from build123d import *

# Parameters (mm, degrees)
CROQUIS1_W              = 250
CROQUIS1_H              = 20
SALIENTE_EXTRUIR1_DEPTH = 250
CROQUIS2_R              = 3.25
CORTAR_EXTRUIR1_DEPTH   = 281.223125384


with BuildPart() as part:
    # Croquis1 → Saliente-Extruir1 (new body)
    with BuildSketch(Plane(origin=(0, 0, 0), x_dir=(1, 0, 0), z_dir=(0, 1, 0))):
        with Locations((0, 185.6)):
            Rectangle(CROQUIS1_W, CROQUIS1_H)
    extrude(amount=SALIENTE_EXTRUIR1_DEPTH)

    # Croquis2 → Cortar-Extruir1 (cut, through all)
    with BuildSketch(Plane.XY.offset(-175.6)):
        with Locations((-77, 21)):
            Circle(CROQUIS2_R)
        with Locations(Location((77, 21, 0), (0, 0, 180))):
            Circle(CROQUIS2_R)
    extrude(amount=-CORTAR_EXTRUIR1_DEPTH, mode=Mode.SUBTRACT)


solid = part.part
For this review, take the finished solid that the model builds, in its own axes (mm). Coordinates: 2 decimals unless noted, no trailing zeros. Loops run counter-clockwise (first coordinate to the right, second up) from the corner with the lowest first, then second, coordinate; pieces in that order, holes last. Notation, with made-up numbers: (43, 7) - (90, 7) arc R20 ccw to (90, 44) - close; hole circle Ø9 at (-28.75, -14.5). An arc over 180 degrees is marked (long way). Return JSON: item names as keys, results as strings.
Item 1: Mouldability with a two-part tool opening along X and no side actions: class faces 1 (the flat face through (-2, 123, -175.6)), 2 (the cylindrical face through (-80.247, 21.143, -185.46)), 3 (the flat face through (-125, 123, -185)) as pulls with the +X half, pulls with the -X half, needs draft (parallel to the pull), parting line crosses it, or undercut.
Determined:
{"face 1": "needs draft", "face 2": "undercut", "face 3": "pulls with the -X half"}
Item 2: Take a section at A-A (x = -77). Give the boundary of the cut face in (y, z), then the cut area to 3 significant figures.
Determined:
{"outline": "(0, -195.6) - (17.75, -195.6) - (17.75, -175.6) - (0, -175.6) - close; (24.25, -195.6) - (250, -195.6) - (250, -175.6) - (24.25, -175.6) - close", "area": "4,870 mm2"}
Item 3: For line 1 (Y direction, x = -77, z = -189), list the stretches that pass through material, from the lowest coordinate up.
Determined:
{"line 1": "y = 0 to 17.75, 24.25 to 250"}
Item 4: Take a section at B-B (y = 21). Give the boundary of the cut face in (x, z), then the cut area to 3 significant figures.
Determined:
{"outline": "(-125, -195.6) - (-80.25, -195.6) - (-80.25, -175.6) - (-125, -175.6) - close; (-73.75, -195.6) - (73.75, -195.6) - (73.75, -175.6) - (-73.75, -175.6) - close; (80.25, -195.6) - (125, -195.6) - (125, -175.6) - (80.25, -175.6) - close", "area": "4,740 mm2"}
